from build123d import *

# Parameters (mm, degrees)
SKETCH1_W                   = 31.75
SKETCH1_H                   = 12.7
BOSS_EXTRUDE1_DEPTH         = 12.7
F_1_4_20_TAPPED_HOLE1_D     = 5.1054
F_1_4_20_TAPPED_HOLE1_DEPTH = 16.51
F_1_4_20_TAPPED_HOLE1_TIP   = 1.533816902
SKETCH4_R                   = 3.3782
CUT_EXTRUDE1_DEPTH          = 13.7


with BuildPart() as part:
    # Sketch1 → Boss-Extrude1 (new body)
    with BuildSketch(Plane(origin=(0, 0, 0), x_dir=(0, 0, -1), z_dir=(1, 0, 0))):
        with Locations((15.875, 6.35)):
            Rectangle(SKETCH1_W, SKETCH1_H)
    extrude(amount=BOSS_EXTRUDE1_DEPTH)

    # 1/4-20 Tapped Hole1
    with Locations(Plane.XY):
        with Locations((6.35, 6.35)):
            Hole(F_1_4_20_TAPPED_HOLE1_D / 2, depth=F_1_4_20_TAPPED_HOLE1_DEPTH)
            with Locations((0, 0, -(F_1_4_20_TAPPED_HOLE1_DEPTH + F_1_4_20_TAPPED_HOLE1_TIP / 2))):  # 118° drill point
                Cone(0, F_1_4_20_TAPPED_HOLE1_D / 2, F_1_4_20_TAPPED_HOLE1_TIP, mode=Mode.SUBTRACT)

    # Sketch4 → Cut-Extrude1 (cut, through all)
    with BuildSketch(Plane(origin=(12.7, 0, 0), x_dir=(0, 0, -1), z_dir=(1, 0, 0))):
        with Locations((25.4, 6.35)):
            Circle(SKETCH4_R)
    extrude(amount=-CUT_EXTRUDE1_DEPTH, mode=Mode.SUBTRACT)


solid = part.part
For this review, take the finished solid that the model builds, in its own axes (mm). A direction names the side the tool comes from. Round coordinates to 2 decimals unless told otherwise and drop trailing zeros. Loops run counter-clockwise (first coordinate to the right, second up) from the corner with the lowest first, then second, coordinate; pieces in that order, holes last. Notation, with made-up numbers: (5.25, 12) - (61.25, 12) arc R24 cw to (61.25, 31) - close; hole circle Ø2 at (3, -24). An arc over 180 degrees is marked (long way). Put each result on its own line as item: value. Start each with the question number.
1. For probe 1 along Y at (x, z) = (6.35, -5.75); probe 2 along Y at (x, z) = (9, -25.4), list the stretches that pass through material, from the lowest coordinate up. Write a range as [from, to].
2. Consider section A-A on z = -25.4. State the section outline as (x, y) points, plus the area to 3 significant figures.
3. Consider section B-B on y = 9.25. State the section outline as (x, z) points.
4. Consider section D-D on z = -5.5. State the section outline as (x, y) points, plus the area to 3 significant figures.
5. For faces 1 (the flat face through (12.7, 6, -16)), 2 (the cylindrical face through (5.172, 4.085, -8.371)), list the 3-axis set-ups (+Z, -Z, +X, -X, +Y, -Y) from which the entire face can be reached by the end or side of a thin tool; tool diameter is ignored.
6. Consider section C-C on x = 10.5. State the section outline as (y, z) points, plus the area to 3 significant figures.
7. Mouldability with a two-part tool opening along Y and no side actions: class faces 3 (the flat face through (6, 12.7, -16)), 4 (the flat face through (0, 6, -16)), 5 (the cylindrical face through (6.439, 6.499, -22.025)), 6 (the conical face through (6.59, 6.72, -17.78)) as +Y half, -Y half, draft (parallel to the pull), parting line (faces both ways), or undercut.
Result sheet:
1. probe 1: [0, 3.8], [8.9, 12.7]
1. probe 2: [0, 2.97], [9.73, 12.7]
2. outline: (0, 0) - (12.7, 0) - (12.7, 2.97) - (0, 2.97) - close; (0, 9.73) - (12.7, 9.73) - (12.7, 12.7) - (0, 12.7) - close
2. area: 75.5 mm^2
3. outline: (0, -31.75) - (12.7, -31.75) - (12.7, -27.13) - (0, -27.13) - close; (0, -23.67) - (12.7, -23.67) - (12.7, 0) - (0, 0) - close
4. outline: (0, 0) - (12.7, 0) - (12.7, 12.7) - (0, 12.7) - close; hole circle Ø5.11 at (6.35, 6.35)
4. area: 141 mm^2
5. face 1: +Z, -Z, +X, +Y, -Y
5. face 2: +Z
6. outline: (0, -31.75) - (12.7, -31.75) - (12.7, 0) - (0, 0) - close; hole circle Ø6.76 at (6.35, -25.4)
6. area: 367 mm^2
7. face 3: +Y half
7. face 4: draft
7. face 5: undercut
7. face 6: undercut
